Check sheet for the modelled part. Datum: model origin and axes. Units: mm. Coordinates: 2 decimals unless noted, no trailing zeros. Use a Markdown table: item, result. Add a question column.
1) Sectioned sample at A-A, the plane y = 2. State how many separate pieces and enclosed holes the cut face has, then the cut area to 3 significant figures.
2) Thickness scan on line 1 (Z direction, x = 52.3, y = 1.05); line 2 (Z direction, x = 38.5, y = 0.4); line 3 (Z direction, x = -30, y = 2.3). Record the ranges inside material, lowest first.
3) Go/stop test with a flat-tipped pin: P1, Ø4.5, axis at x = 10, z = 40, coming from the +Y side. Record where the tip stops, or that it passes through.
from build123d import *

# Parameters (mm, degrees)
SKETCH1_R           = 3.55
SKETCH1_R_2         = 2.6
BOSS_EXTRUDE1_DEPTH = 3


with BuildPart() as part:
    # Sketch1 → Boss-Extrude1 (new body)
    with BuildSketch(Plane(origin=(0, 0, 0), x_dir=(1, 0, 0), z_dir=(0, 1, 0))):
        with BuildLine():
            Line((60, -80), (-60, -80))
            ThreePointArc((-60, -80), (-67.071067812, -77.071067812), (-70, -70))
            Line((-70, -70), (-70, 70))
            ThreePointArc((-70, 70), (-67.071067812, 77.071067812), (-60, 80))
            Line((-60, 80), (60, 80))
            ThreePointArc((60, 80), (67.071067812, 77.071067812), (70, 70))
            Line((70, 70), (70, -70))
            ThreePointArc((70, -70), (67.071067812, -77.071067812), (60, -80))
        make_face()
        with Locations((-42.3, 62.3)):
            Circle(SKETCH1_R, mode=Mode.SUBTRACT)
        with Locations((0, 10)):
            Circle(SKETCH1_R_2, mode=Mode.SUBTRACT)
        Circle(SKETCH1_R_2, mode=Mode.SUBTRACT)
        with Locations((10, 0)):
            Circle(SKETCH1_R_2, mode=Mode.SUBTRACT)
        with Locations((-10, 0)):
            Circle(SKETCH1_R_2, mode=Mode.SUBTRACT)
        with Locations((-52.3, 62.3)):
            Circle(SKETCH1_R, mode=Mode.SUBTRACT)
        with Locations((-52.3, 0)):
            Circle(SKETCH1_R, mode=Mode.SUBTRACT)
        with Locations((-52.3, -62.3)):
            Circle(SKETCH1_R, mode=Mode.SUBTRACT)
        with Locations((-40, 30)):
            Circle(SKETCH1_R_2, mode=Mode.SUBTRACT)
        with Locations((-40, 10)):
            Circle(SKETCH1_R_2, mode=Mode.SUBTRACT)
        with Locations((-30, 40)):
            Circle(SKETCH1_R_2, mode=Mode.SUBTRACT)
        with Locations((0, 30)):
            Circle(SKETCH1_R_2, mode=Mode.SUBTRACT)
        with Locations((-10, 62.3)):
            Circle(SKETCH1_R_2, mode=Mode.SUBTRACT)
        with Locations((0, 62.3)):
            Circle(SKETCH1_R_2, mode=Mode.SUBTRACT)
        with Locations((10, 62.3)):
            Circle(SKETCH1_R_2, mode=Mode.SUBTRACT)
        with Locations((-10, 40)):
            Circle(SKETCH1_R_2, mode=Mode.SUBTRACT)
        with Locations((30, 40)):
            Circle(SKETCH1_R_2, mode=Mode.SUBTRACT)
        with Locations((40, 30)):
            Circle(SKETCH1_R_2, mode=Mode.SUBTRACT)
        with Locations((40, 10)):
            Circle(SKETCH1_R_2, mode=Mode.SUBTRACT)
        with Locations((42.3, 62.3)):
            Circle(SKETCH1_R_2, mode=Mode.SUBTRACT)
        with Locations((52.3, 62.3)):
            Circle(SKETCH1_R_2, mode=Mode.SUBTRACT)
        with Locations((52.3, 0)):
            Circle(SKETCH1_R_2, mode=Mode.SUBTRACT)
        with Locations((40, -10)):
            Circle(SKETCH1_R_2, mode=Mode.SUBTRACT)
        with Locations((52.3, -62.3)):
            Circle(SKETCH1_R_2, mode=Mode.SUBTRACT)
        with Locations((42.3, -62.3)):
            Circle(SKETCH1_R_2, mode=Mode.SUBTRACT)
        with Locations((40, -30)):
            Circle(SKETCH1_R_2, mode=Mode.SUBTRACT)
        with Locations((0, -10)):
            Circle(SKETCH1_R_2, mode=Mode.SUBTRACT)
        with Locations((30, -40)):
            Circle(SKETCH1_R_2, mode=Mode.SUBTRACT)
        with Locations((10, 40)):
            Circle(SKETCH1_R_2, mode=Mode.SUBTRACT)
        with Locations((10, -62.3)):
            Circle(SKETCH1_R_2, mode=Mode.SUBTRACT)
        with Locations((0, -62.3)):
            Circle(SKETCH1_R_2, mode=Mode.SUBTRACT)
        with Locations((-10, -62.3)):
            Circle(SKETCH1_R_2, mode=Mode.SUBTRACT)
        with Locations((30, 0)):
            Circle(SKETCH1_R_2, mode=Mode.SUBTRACT)
        with Locations((-30, -40)):
            Circle(SKETCH1_R_2, mode=Mode.SUBTRACT)
        with Locations((-40, -30)):
            Circle(SKETCH1_R_2, mode=Mode.SUBTRACT)
        with Locations((-40, -10)):
            Circle(SKETCH1_R_2, mode=Mode.SUBTRACT)
        with Locations((-42.3, -62.3)):
            Circle(SKETCH1_R, mode=Mode.SUBTRACT)
        with Locations((-32.3, 62.3)):
            Circle(SKETCH1_R, mode=Mode.SUBTRACT)
        with Locations((32.3, 62.3)):
            Circle(SKETCH1_R_2, mode=Mode.SUBTRACT)
        with Locations((22.3, -62.3)):
            Circle(SKETCH1_R_2, mode=Mode.SUBTRACT)
        with Locations((-30, 0)):
            Circle(SKETCH1_R_2, mode=Mode.SUBTRACT)
        with Locations((-52.3, 35)):
            Circle(SKETCH1_R, mode=Mode.SUBTRACT)
        with Locations((32.3, -62.3)):
            Circle(SKETCH1_R_2, mode=Mode.SUBTRACT)
        with Locations((-32.3, -62.3)):
            Circle(SKETCH1_R, mode=Mode.SUBTRACT)
        with Locations((-52.3, -35)):
            Circle(SKETCH1_R, mode=Mode.SUBTRACT)
        with Locations((52.3, 35)):
            Circle(SKETCH1_R_2, mode=Mode.SUBTRACT)
        with Locations((52.3, -35)):
            Circle(SKETCH1_R_2, mode=Mode.SUBTRACT)
        with Locations((-22.3, 62.3)):
            Circle(SKETCH1_R, mode=Mode.SUBTRACT)
        with Locations((22.3, 62.3)):
            Circle(SKETCH1_R_2, mode=Mode.SUBTRACT)
        with Locations((-22.3, -62.3)):
            Circle(SKETCH1_R, mode=Mode.SUBTRACT)
        with Locations((10, -40)):
            Circle(SKETCH1_R_2, mode=Mode.SUBTRACT)
        with Locations((-10, -40)):
            Circle(SKETCH1_R_2, mode=Mode.SUBTRACT)
        with Locations((0, -30)):
            Circle(SKETCH1_R_2, mode=Mode.SUBTRACT)
        with Locations((-55, 10)):
            Circle(SKETCH1_R_2, mode=Mode.SUBTRACT)
        with Locations((55, 10)):
            Circle(SKETCH1_R_2, mode=Mode.SUBTRACT)
        with Locations((55, -10)):
            Circle(SKETCH1_R_2, mode=Mode.SUBTRACT)
        with Locations((-55, -10)):
            Circle(SKETCH1_R_2, mode=Mode.SUBTRACT)
    extrude(amount=BOSS_EXTRUDE1_DEPTH)


solid = part.part
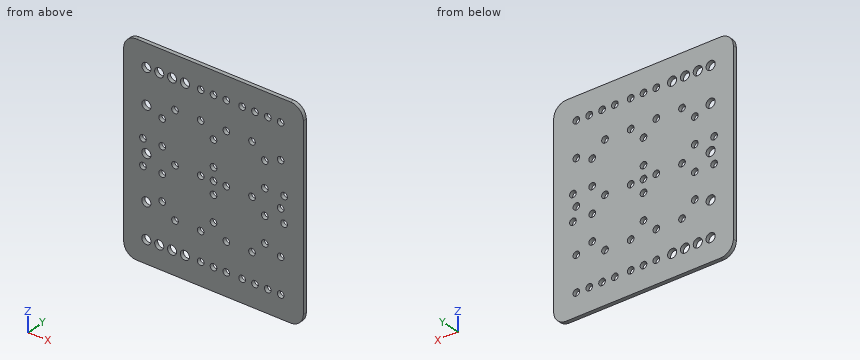
Solved:
| question | item | result |
|---|---|---|
| 1 | separate pieces | 1 |
| 1 | enclosed holes | 57 |
| 1 | area | 20,900 mm2 |
| 2 | line 1 | z = -80 to -64.9, -59.7 to -37.6, -32.4 to -2.6, 2.6 to 32.4, 37.6 to 59.7, 64.9 to 80 |
| 2 | line 2 | z = -80 to -32.12, -27.88 to -12.12, -7.88 to 7.88, 12.12 to 27.88, 32.12 to 80 |
| 2 | line 3 | z = -80 to -65, -59.6 to -42.6, -37.4 to -2.6, 2.6 to 37.4, 42.6 to 59.6, 65 to 80 |
| 3 | P1 | passes through |
